```python
from build123d import *

# Parameters (mm, degrees)
SKETCH_1_W          = 9
SKETCH_1_H          = 250
EXTRUDE_1_DEPTH     = 6.5
SKETCH_2_R          = 1.6
CUT_EXTRUDE_1_DEPTH = 126.249750499
SKETCH_3_R          = 3.25
CUT_EXTRUDE_2_DEPTH = 3


with BuildPart() as part:
    # 草图1 → 凸台-拉伸1 (new body)
    with BuildSketch(Plane.XY):
        Rectangle(SKETCH_1_W, SKETCH_1_H)
    extrude(amount=EXTRUDE_1_DEPTH)

    # 草图2 → 切除-拉伸1 (cut, through all)
    with BuildSketch(Plane.XY.offset(6.5)):
        Circle(SKETCH_2_R)
        with Locations((0, 20)):
            Circle(SKETCH_2_R)
        with Locations((0, 40)):
            Circle(SKETCH_2_R)
        with Locations((0, 60)):
            Circle(SKETCH_2_R)
        with Locations((0, 80)):
            Circle(SKETCH_2_R)
        with Locations((0, -20)):
            Circle(SKETCH_2_R)
        with Locations((0, -40)):
            Circle(SKETCH_2_R)
        with Locations((0, -60)):
            Circle(SKETCH_2_R)
        with Locations((0, -80)):
            Circle(SKETCH_2_R)
    extrude(amount=-CUT_EXTRUDE_1_DEPTH, mode=Mode.SUBTRACT)

    # 草图3 → 切除-拉伸2 (cut)
    with BuildSketch(Plane.XY.offset(6.5)):
        with Locations((0, 80)):
            Circle(SKETCH_3_R)
        with Locations((0, 60)):
            Circle(SKETCH_3_R)
        with Locations((0, 40)):
            Circle(SKETCH_3_R)
        with Locations((0, 20)):
            Circle(SKETCH_3_R)
        Circle(SKETCH_3_R)
        with Locations((0, -20)):
            Circle(SKETCH_3_R)
        with Locations((0, -40)):
            Circle(SKETCH_3_R)
        with Locations((0, -60)):
            Circle(SKETCH_3_R)
        with Locations((0, -80)):
            Circle(SKETCH_3_R)
    extrude(amount=-CUT_EXTRUDE_2_DEPTH, mode=Mode.SUBTRACT)


solid = part.part
```
Geometry check sheet. Reference: the model listing, model coordinates, mm. A direction names the side the tool comes from. Give positions to 0.01 mm unless a question says otherwise; leave off trailing zeros. Answer as CSV lines item,"result".
Item 1: Depth check by flat-ended pin: P1, Ø5, axis at x = 0, y = -60.5, coming from the +Z side; P2, Ø3, axis at x = 0, y = 0, coming from the +Z side. Enter the tip coordinate at first touch or a pass-through.
Values:
P1,"stops at z = 3.5"
P2,"passes through"
Item 2: Cross-section at A-A on z = 2. Count the separate pieces of the cut face and the enclosed holes in it, and give its area (3 significant figures).
Values:
separate pieces,"1"
enclosed holes,"9"
area,"2,180 mm²"
Item 3: Material ranges on line 1 (Z direction, x = 2.25, y = -62), recorded low to high.
Values:
line 1,"z = 0 to 3.5"
Item 4: Release check for a two-part mould opening along Y. For faces 3 (the flat face through (-4.5, -2, 3)), 4 (the flat face through (0, -125, 3)), 5 (the flat face through (1.4, 58.6, 3.5)), 6 (the flat face through (1.4, -41.4, 3.5)) record: pulls with the +Y half, pulls with the -Y half, needs draft (parallel to the pull), parting line crosses it, or undercut.
Values:
face 3,"needs draft"
face 4,"pulls with the -Y half"
face 5,"undercut"
face 6,"undercut"
Item 5: Access from +Z, -Z, +X, -X, +Y, -Y to the whole of each face (thin tool, end or side, straight path). Record for faces 1 (the flat face through (1.4, 38.6, 3.5)), 2 (the flat face through (4.5, -2, 3)).
Values:
face 1,"+Z"
face 2,"+Z, -Z, +X, +Y, -Y"
